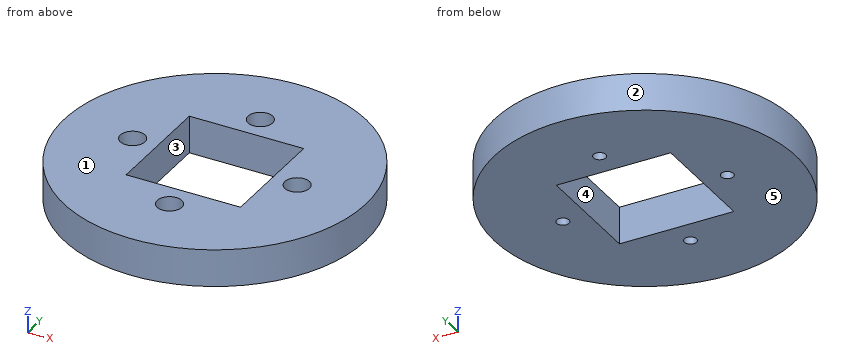
```python
from build123d import *

# Parameters (mm, degrees)
SKETCH1_R           = 40.3
SKETCH1_R_2         = 1.65
SKETCH1_W           = 30.6
SKETCH1_H           = 30.6
BOSS_EXTRUDE1_DEPTH = 10
SKETCH2_R           = 3.3
CUT_EXTRUDE1_DEPTH  = 6


with BuildPart() as part:
    # Sketch1 → Boss-Extrude1 (new body)
    with BuildSketch(Plane.XY):
        Circle(SKETCH1_R)
        with Locations((0, 22)):
            Circle(SKETCH1_R_2, mode=Mode.SUBTRACT)
        with Locations((22, 0)):
            Circle(SKETCH1_R_2, mode=Mode.SUBTRACT)
        with Locations((0, -22)):
            Circle(SKETCH1_R_2, mode=Mode.SUBTRACT)
        with Locations((-22, 0)):
            Circle(SKETCH1_R_2, mode=Mode.SUBTRACT)
        Rectangle(SKETCH1_W, SKETCH1_H, mode=Mode.SUBTRACT)
    extrude(amount=BOSS_EXTRUDE1_DEPTH)

    # Sketch2 → Cut-Extrude1 (cut)
    with BuildSketch(Plane.XY.offset(10)):
        with Locations((22, 0)):
            Circle(SKETCH2_R)
        with Locations((0, 22)):
            Circle(SKETCH2_R)
        with Locations((-22, 0)):
            Circle(SKETCH2_R)
        with Locations((0, -22)):
            Circle(SKETCH2_R)
    extrude(amount=-CUT_EXTRUDE1_DEPTH, mode=Mode.SUBTRACT)


solid = part.part
```
Work out the finished part from the listing and answer in its coordinate system (mm). Face numbers are marked on the shaded views. A direction names the side the tool comes from. Round coordinates to 2 decimals unless told otherwise and drop trailing zeros. Write each loop counter-clockwise with the first axis right and the second up, starting at its lowest first coordinate (ties: lowest second). Pieces come first, ordered by that corner, then holes.
1) Determine the mould class of the marked faces 1, 2 and 3 for opening direction X: pulls with the +X half, pulls with the -X half, needs draft (parallel to the pull), parting line crosses it, or undercut.
2) A cutting plane is placed at A-A on y = 0. Determine the outline of the cut face in (x, z), and give its area (3 significant figures).
3) A cutting plane is placed at D-D on y = 22. Determine the outline of the cut face in (x, z).
4) A cutting plane is placed at C-C on z = 8.75. Determine the outline of the cut face in (x, y), and give its area (3 significant figures).
5) Flat-ended cylindrical pins translate along their axes: P1, Ø3, axis at x = -7, z = 8.5, coming from the +Y side; P2, Ø3, axis at x = 22, y = 0, coming from the +Z side; P3, Ø4, axis at y = -6.5, z = 2, coming from the -X side; P4, Ø4, axis at x = -22, y = 0, coming from the +Z side. Find the tip coordinate at first contact, or state that the pin passes through.
6) Which of the six approach directions +Z, -Z, +X, -X, +Y, -Y give full straight-line access (tool end or side, diameter ignored) to the marked faces 4 and 5?
7) Consider probe 1 along Y at (x, z) = (0, 7.05); probe 2 along Y at (x, z) = (1, 5); probe 3 along Y at (x, z) = (14, 1). Determine where each line is inside the solid, lowest interval first.
Entries:
1. face 1: needs draft
1. face 2: parting line crosses it
1. face 3: undercut
2. outline: (-40.3, 0) - (-23.65, 0) - (-23.65, 4) - (-25.3, 4) - (-25.3, 10) - (-40.3, 10) - close; (-20.35, 0) - (-15.3, 0) - (-15.3, 10) - (-18.7, 10) - (-18.7, 4) - (-20.35, 4) - close; (15.3, 0) - (20.35, 0) - (20.35, 4) - (18.7, 4) - (18.7, 10) - (15.3, 10) - close; (23.65, 0) - (40.3, 0) - (40.3, 10) - (25.3, 10) - (25.3, 4) - (23.65, 4) - close
2. area: 394 mm2
3. outline: (-33.77, 0) - (-1.65, 0) - (-1.65, 4) - (-3.3, 4) - (-3.3, 10) - (-33.77, 10) - close; (1.65, 0) - (33.77, 0) - (33.77, 10) - (3.3, 10) - (3.3, 4) - (1.65, 4) - close
4. outline: circle Ø80.6 at (0, 0); hole circle Ø6.6 at (-22, 0); hole (-15.3, -15.3) - (15.3, -15.3) - (15.3, 15.3) - (-15.3, 15.3) - close; hole circle Ø6.6 at (0, -22); hole circle Ø6.6 at (0, 22); hole circle Ø6.6 at (22, 0)
4. area: 4,030 mm2
5. P1: stops at y = 39.92
5. P2: passes through
5. P3: stops at x = -40.05
5. P4: stops at z = 4
6. face 4: +Z, -Z
6. face 5: -Z, +X, -X, +Y, -Y
7. probe 1: y = -40.3 to -25.3, -18.7 to -15.3, 15.3 to 18.7, 25.3 to 40.3
7. probe 2: y = -40.29 to -25.14, -18.86 to -15.3, 15.3 to 18.86, 25.14 to 40.29
7. probe 3: y = -37.79 to -15.3, 15.3 to 37.79
